Geometry: final body of the model. Coordinates: model frame, mm. A direction names the side the tool comes from. Give positions to 0.01 mm unless a question says otherwise; leave off trailing zeros. Loops run counter-clockwise (first coordinate to the right, second up) from the corner with the lowest first, then second, coordinate; pieces in that order, holes last.
1. Section A-A, the plane x = 6.5. Output: boundary loops of the cut face in (y, z) (3 decimals).
2. Access query for faces 1 (the face through (10.77, 1.93, -7.48)), 2 (the face through (4, 2, -20.51)). Directions: +Z, -Z, +X, -X, +Y, -Y. A direction counts if a zero-diameter tool reaches every point of the face in a straight line with its end or side. Return the directions, or none.
3. Section D-D, the plane z = -6.75. Output: boundary loops of the cut face in (x, y).
4. Draft query along Z for faces 3 (the face through (20.066, 2, -17)), 4 (the face through (13, 2, -25.4)), 5 (the face through (13, 3.81, -13)). Return one class per face: +Z half, -Z half, draft (parallel to the pull), parting line (faces both ways), or undercut.
5. Material intervals for line 1 along X through (y, z) = (0.45, -17); line 2 along Z through (x, y) = (4.75, 1.65); line 3 along X through (y, z) = (1.4, -5.25), sorted ascending.
6. Section C-C, the plane y = 0.5. State how many separate pieces and enclosed holes the cut face has, then the cut area to 3 significant figures.
7. Section B-B, the plane z = -17.5. Output: boundary loops of the cut face in (x, y).
from build123d import *

# Parameters (mm, degrees)
BOSS_EXTRUDE1_DEPTH = 3.81
CUT_EXTRUDE1_DEPTH  = 37.122515139
SKETCH4_W           = 2.413
SKETCH4_H           = 1.27
CUT_EXTRUDE2_DEPTH  = 2.2352
SKETCH6_W           = 2.413
SKETCH6_H           = 1.27
CUT_EXTRUDE3_DEPTH  = 2.2352


with BuildPart() as part:
    # Sketch1 → Boss-Extrude1 (new body)
    with BuildSketch(Plane(origin=(0, 0, 0), x_dir=(1, 0, 0), z_dir=(0, 1, 0))):
        with BuildLine():
            Line((0.635, 0), (24.765, 0))
            ThreePointArc((24.765, 0), (25.214012806, 0.185987194), (25.4, 0.635))
            Line((25.4, 0.635), (25.4, 24.765))
            ThreePointArc((25.4, 24.765), (25.214012806, 25.214012806), (24.765, 25.4))
            Line((24.765, 25.4), (0.635, 25.4))
            ThreePointArc((0.635, 25.4), (0.185987194, 25.214012806), (0, 24.765))
            Line((0, 24.765), (0, 0.635))
            ThreePointArc((0, 0.635), (0.185987194, 0.185987194), (0.635, 0))
        make_face()
    extrude(amount=BOSS_EXTRUDE1_DEPTH)

    # Sketch2 → Cut-Extrude1 (cut, through all)
    with BuildSketch(Plane(origin=(0, 3.81, 0), x_dir=(1, 0, 0), z_dir=(0, 1, 0))):
        with BuildLine():
            Line((10.1346, 2.8194), (15.2654, 2.8194))
            ThreePointArc((15.2654, 2.8194), (15.355202561, 2.856597439), (15.3924, 2.9464))
            Line((15.3924, 2.9464), (15.3924, 5.6642))
            ThreePointArc((15.3924, 5.6642), (14.648451224, 7.460251224), (12.8524, 8.2042))
            Line((12.8524, 8.2042), (12.5476, 8.2042))
            ThreePointArc((12.5476, 8.2042), (10.751548776, 7.460251224), (10.0076, 5.6642))
            Line((10.0076, 5.6642), (10.0076, 2.9464))
            ThreePointArc((10.0076, 2.9464), (10.044797439, 2.856597439), (10.1346, 2.8194))
        make_face()
        with BuildLine():
            Line((5.461, 20.955), (7.239, 20.955))
            ThreePointArc((7.239, 20.955), (7.328802561, 20.917802561), (7.366, 20.828))
            Line((7.366, 20.828), (7.366, 13.97))
            ThreePointArc((7.366, 13.97), (7.328802561, 13.880197439), (7.239, 13.843))
            Line((7.239, 13.843), (5.461, 13.843))
            ThreePointArc((5.461, 13.843), (5.371197439, 13.880197439), (5.334, 13.97))
            Line((5.334, 13.97), (5.334, 14.2875))
            Line((5.334, 14.2875), (5.334, 16.7005))
            Line((5.334, 16.7005), (5.334, 18.0975))
            Line((5.334, 18.0975), (5.334, 20.5105))
            Line((5.334, 20.5105), (5.334, 20.828))
            ThreePointArc((5.334, 20.828), (5.371197439, 20.917802561), (5.461, 20.955))
        make_face()
        with BuildLine():
            Line((18.161, 21.844), (19.939, 21.844))
            ThreePointArc((19.939, 21.844), (20.028802561, 21.806802561), (20.066, 21.717))
            Line((20.066, 21.717), (20.066, 20.5105))
            Line((20.066, 20.5105), (20.066, 18.0975))
            Line((20.066, 18.0975), (20.066, 16.7005))
            Line((20.066, 16.7005), (20.066, 14.2875))
            Line((20.066, 14.2875), (20.066, 13.081))
            ThreePointArc((20.066, 13.081), (20.028802561, 12.991197439), (19.939, 12.954))
            Line((19.939, 12.954), (18.161, 12.954))
            ThreePointArc((18.161, 12.954), (18.071197439, 12.991197439), (18.034, 13.081))
            Line((18.034, 13.081), (18.034, 21.717))
            ThreePointArc((18.034, 21.717), (18.071197439, 21.806802561), (18.161, 21.844))
        make_face()
    extrude(amount=-CUT_EXTRUDE1_DEPTH, mode=Mode.SUBTRACT)

    # Sketch4 → Cut-Extrude2 (cut)
    with BuildSketch(Plane(origin=(5.334, 0, 0), x_dir=(0, 0, -1), z_dir=(1, 0, 0))):
        with Locations((15.494, 1.905)):
            Rectangle(SKETCH4_W, SKETCH4_H)
        with Locations((19.304, 1.905)):
            Rectangle(SKETCH4_W, SKETCH4_H)
    extrude(amount=-CUT_EXTRUDE2_DEPTH, mode=Mode.SUBTRACT)

    # Sketch6 → Cut-Extrude3 (cut)
    with BuildSketch(Plane.ZY.offset(-20.066)):
        with Locations((-15.494, 1.905)):
            Rectangle(SKETCH6_W, SKETCH6_H)
        with Locations((-19.304, 1.905)):
            Rectangle(SKETCH6_W, SKETCH6_H)
    extrude(amount=-CUT_EXTRUDE3_DEPTH, mode=Mode.SUBTRACT)


solid = part.part
Answers below:
1. outline: (0, -25.4) - (3.81, -25.4) - (3.81, -20.955) - (0, -20.955) - close; (0, -13.843) - (3.81, -13.843) - (3.81, 0) - (0, 0) - close
2. face 1: +Y, -Y
2. face 2: none
3. outline: (0, 0) - (10.25, 0) - (10.25, 3.81) - (0, 3.81) - close; (15.15, 0) - (25.4, 0) - (25.4, 3.81) - (15.15, 3.81) - close
4. face 3: undercut
4. face 4: -Z half
4. face 5: draft
5. line 1: x = 0 to 5.33, 7.37 to 18.03, 20.07 to 25.4
5. line 2: z = -25.4 to -20.51, -18.1 to -16.7, -14.29 to 0
5. line 3: x = 0 to 10.01, 15.39 to 25.4
6. separate pieces: 1
6. enclosed holes: 3
6. area: 586 mm2
7. outline: (0, 0) - (5.33, 0) - (5.33, 3.81) - (0, 3.81) - close; (7.37, 0) - (18.03, 0) - (18.03, 3.81) - (7.37, 3.81) - close; (20.07, 0) - (25.4, 0) - (25.4, 3.81) - (20.07, 3.81) - close
